The listing builds one solid part. Answer for the finished solid, in the listing's coordinates (mm). A direction names the side the tool comes from. Give positions to 0.01 mm unless a question says otherwise; leave off trailing zeros. Loops run counter-clockwise (first coordinate to the right, second up) from the corner with the lowest first, then second, coordinate; pieces in that order, holes last. Notation, with made-up numbers: M 77,-24.75 L 115,-24.75 A11 ccw 115,-17.75 Z; hole C 48,89.25 d5. An arc over 180 degrees is marked long. Use one line per item in the form item = value. Start each with the question number.
1. For faces 1 (the face through (15.33, 206.57, 8.41)), 2 (the face through (-41.931, -158.634, 1.493)), 3 (the face through (7, -16, 0)), 4 (the face through (177.644, -18.547, 8.409)), 5 (the face through (9, 42, 15)), determine the directions among +Z, -Z, +X, -X, +Y, -Y from which every point of the face is accessible in a straight line to the end or side of a thin tool.
2. Straight lines are drawn through the part: line 1 (Z direction, x = 213, y = 63.5); line 2 (Y direction, x = -102, z = 10.25); line 3 (Y direction, x = -31, z = 3.25). For each, find the intervals that lie inside material, in ascending order. Write a range as from..to.
3. The part is cut by section C-C (z = 6.5). Write down the section's boundary in (x, y), and give its area (3 significant figures).
4. The part is cut by section A-A (y = 15). Write down the section's boundary in (x, z), and give its area (3 significant figures).
5. Each of these flat-tipped pins is pushed along its axis until it touches: pin 1 Ø2 at (y, z) = (-65.5, 10) entering from +X; pin 2 Ø2 at (x, y) = (9.5, 139) entering from -Z; pin 3 Ø1.5 at (y, z) = (-94, 2) entering from +X; pin 4 Ø2 at (y, z) = (161.5, 6) entering from -X. Where does it stop, or does it pass through?
6. The part is cut by section D-D (x = 261.5). Write down the section's boundary in (y, z).
7. The part is cut by section B-B (x = 99). Write down the section's boundary in (y, z), and give its area (3 significant figures).
from build123d import *

# Parameters (mm, degrees)
F0_W     = 600
F0_H     = 600
F5_DEPTH = 1
F1_DEPTH = 2
F2_DEPTH = 15


with BuildPart() as f5:
    # F0 (on Top) → F5 (new body)
    with BuildSketch(Plane.XY):
        with Locations((10.792556, -20.516564)):
            Rectangle(F0_W, F0_H)
        Polygon((-221.498368, 192.184042), (246.932485, 230.557681), (119.79194, -263.340367), (-199.188834, -56.818538), align=None, mode=Mode.SUBTRACT)
    extrude(amount=F5_DEPTH)

    # F0 (on Top) → F1 (join)
    with BuildSketch(Plane.XY):
        Polygon((119.79194, -263.340367), (246.932485, 230.557681), (-221.498368, 192.184042), (-199.188834, -56.818538), align=None)
        Polygon((240.339008, 225.000797), (116.680786, -255.369601), (-194.426209, -53.945594), (-216.068713, 187.612088), align=None, mode=Mode.SUBTRACT)
    extrude(amount=F1_DEPTH)

    # F0 (on Top) → F2 (join)
    with BuildSketch(Plane.XY):
        Polygon((-194.426209, -53.945594), (116.680786, -255.369601), (240.339008, 225.000797), (-216.068713, 187.612088), align=None)
    extrude(amount=F2_DEPTH)


solid = f5.part
Derived:
q1.face_1 = +Z, -X, +Y
q1.face_2 = +Z, -X, -Y
q1.face_3 = -Z, +X, -X, +Y, -Y
q1.face_4 = +Z, +X, -Y
q1.face_5 = +Z, +X, -X, +Y, -Y
q2.line_1 = 0..1
q2.line_2 = -113.79..196.96
q2.line_3 = -159.75..202.77
q3.outline = M -216.07,187.61 L -194.43,-53.95 L 116.68,-255.37 L 240.34,225 Z
q3.area = 143,000 mm2
q4.outline = M -289.21,0 L 310.79,0 L 310.79,1 L 191.44,1 L 191.44,2 L 186.28,2 L 186.28,15 L -200.6,15 L -200.6,2 L -205.62,2 L -205.62,1 L -289.21,1 Z
q4.area = 6,030 mm2
q5.pin_1 = 165.81
q5.pin_2 = 0
q5.pin_3 = 163.58
q5.pin_4 = -213.82
q6.outline = M -320.52,0 L 279.48,0 L 279.48,1 L -320.52,1 Z
q7.outline = M -320.52,0 L 279.48,0 L 279.48,1 L 218.44,1 L 218.44,2 L 213.42,2 L 213.42,15 L -243.92,15 L -243.92,2 L -249.88,2 L -249.88,1 L -320.52,1 Z
q7.area = 7,010 mm2
